Answer from the drawing. Dimensions are ordinates in mm from the lowest x, y and z of the part. Give positions to 0.01 mm unless a question says otherwise; leave off trailing zeros. Write each question's results on one line, items separated by ' | '.
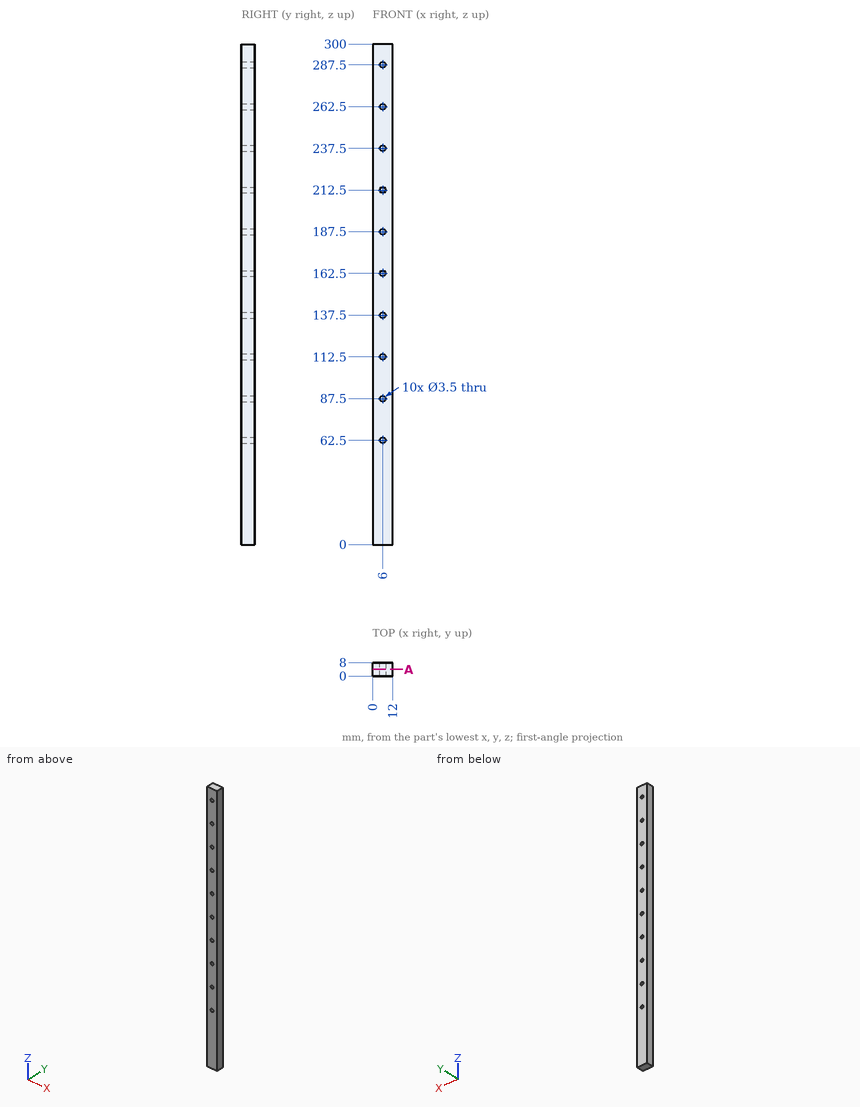
1. A straight line is drawn through the part: line 1 (X direction, y = 4.5, z = 162.5). Find the intervals that lie inside material, in ascending order. Write a range as [from, to].
Answer list:
line 1: [0, 4.25], [7.75, 12]
2. A cutting plane is placed at A-A, the plane y = 4. State how many separate pieces and enclosed holes the cut face has, then the cut area to 3 significant figures.
Answer list:
separate pieces: 1 | enclosed holes: 10 | area: 3,500 mm^2
3. Given P1, Ø3, axis at x = 6, z = 187.5, coming from the +Y side, flat-ended and moving along its own axis, determine where the tip first touches the part or whether it passes through.
Answer list:
P1: through
